For this review, take the finished solid that the model builds, in its own axes (mm). Face numbers are marked on the shaded views. A direction names the side the tool comes from. Round coordinates to 2 decimals unless told otherwise and drop trailing zeros. Write each loop counter-clockwise with the first axis right and the second up, starting at its lowest first coordinate (ties: lowest second). Pieces come first, ordered by that corner, then holes. Notation, with made-up numbers: M 29.5,0.25 L 55.5,0.25 A16 cw 55.5,10.25 Z; hole C -18,27 d5. An arc over 180 degrees is marked long. One line per question, with ' | ' between items.
```python
from build123d import *

# Parameters (mm, degrees)
SKETCH1_W                                       = 140
SKETCH1_H                                       = 30
BOSS_EXTRUDE1_DEPTH                             = 30
SHELL1_T                                        = -5
SKETCH3_W                                       = 5
SKETCH3_H                                       = 20
BOSS_EXTRUDE2_DEPTH                             = 25
SKETCH4_R                                       = 2.5
BOSS_EXTRUDE3_DEPTH                             = 5
SKETCH5_R                                       = 1.5
CUT_EXTRUDE1_DEPTH                              = 20
CUT_EXTRUDE2_DEPTH                              = 152.079449297
CUT_EXTRUDE2_DEPTH_BACK                         = 152.079449297
SKETCH9_R                                       = 5
SKETCH10_W                                      = 140
SKETCH10_H                                      = 5
BOSS_EXTRUDE5_DEPTH                             = 15
SKETCH11_W                                      = 135
SKETCH11_H                                      = 5
CUT_EXTRUDE3_DEPTH                              = 2
FILLET1_R                                       = 2
CSK_FOR_M5_FLAT_HEAD_MACHINE_SCREW1_D           = 5.5
CSK_FOR_M5_FLAT_HEAD_MACHINE_SCREW1_DEPTH       = 20
CSK_FOR_M5_FLAT_HEAD_MACHINE_SCREW1_CSINK_D     = 10.4
CSK_FOR_M5_FLAT_HEAD_MACHINE_SCREW1_CSINK_ANGLE = 90
CSK_FOR_M5_FLAT_HEAD_MACHINE_SCREW1_TIP         = 1.652366702
FILLET2_R                                       = 5


with BuildPart() as part:
    # Sketch1 → Boss-Extrude1 (new body)
    with BuildSketch(Plane(origin=(0, 0, 0), x_dir=(1, 0, 0), z_dir=(0, 1, 0))):
        with Locations((70, 15)):
            Rectangle(SKETCH1_W, SKETCH1_H)
    extrude(amount=BOSS_EXTRUDE1_DEPTH)

    # Shell1
    shell1_openings = [part.faces().sort_by_distance(p)[0] for p in [
        (70, 0, -15),
    ]]
    offset(amount=SHELL1_T, openings=shell1_openings, kind=Kind.INTERSECTION)

    # Sketch3 → Boss-Extrude2 (add)
    with BuildSketch(Plane.XZ.offset(-25)):
        with Locations((52.5, -15)):
            Rectangle(SKETCH3_W, SKETCH3_H)
    extrude(amount=BOSS_EXTRUDE2_DEPTH)

    # Sketch4 → Boss-Extrude3 (add)
    with BuildSketch(Plane(origin=(140, 0, 0), x_dir=(0, 0, -1), z_dir=(1, 0, 0))):
        with Locations(Location((8, 22, 0), (0, 0, 180))):
            Circle(SKETCH4_R)
        with Locations(Location((22, 22, 0), (0, 0, 180))):
            Circle(SKETCH4_R)
        with Locations(Location((8, 8, 0), (0, 0, 180))):
            Circle(SKETCH4_R)
        with Locations(Location((22, 8, 0), (0, 0, 180))):
            Circle(SKETCH4_R)
    extrude(amount=BOSS_EXTRUDE3_DEPTH)

    # Sketch5 → Cut-Extrude1 (cut)
    with BuildSketch(Plane.ZY):
        with Locations((-15, 15)):
            Circle(SKETCH5_R)
    extrude(amount=-CUT_EXTRUDE1_DEPTH, mode=Mode.SUBTRACT)

    # Sketch9 → Cut-Extrude2 (cut, two sides: drawn at the far end of the back side and taken through both)
    with BuildSketch(Plane.XY.offset(-CUT_EXTRUDE2_DEPTH_BACK)):
        with Locations((125, 15)):
            Circle(SKETCH9_R)
    extrude(amount=CUT_EXTRUDE2_DEPTH + CUT_EXTRUDE2_DEPTH_BACK, mode=Mode.SUBTRACT)

    # Sketch10 → Boss-Extrude5 (add)
    with BuildSketch(Plane(origin=(0, 30, 0), x_dir=(1, 0, 0), z_dir=(0, 1, 0))):
        with Locations((70, 17.5)):
            Rectangle(SKETCH10_W, SKETCH10_H)
    extrude(amount=BOSS_EXTRUDE5_DEPTH)

    # Sketch11 → Cut-Extrude3 (cut)
    with BuildSketch(Plane.XY.offset(-15)):
        with Locations((72.5, 37.5)):
            Rectangle(SKETCH11_W, SKETCH11_H)
    extrude(amount=-CUT_EXTRUDE3_DEPTH, mode=Mode.SUBTRACT)

    # Fillet1
    fillet1_edges = [part.edges().sort_by_distance(p)[0] for p in [
        (70, 45, -15),
    ]]
    fillet(fillet1_edges, radius=FILLET1_R)

    # CSK for M5 Flat Head Machine Screw1
    with Locations(Plane.ZY):
        with Locations((-15, 15)):
            CounterSinkHole(CSK_FOR_M5_FLAT_HEAD_MACHINE_SCREW1_D / 2, CSK_FOR_M5_FLAT_HEAD_MACHINE_SCREW1_CSINK_D / 2, depth=CSK_FOR_M5_FLAT_HEAD_MACHINE_SCREW1_DEPTH, counter_sink_angle=CSK_FOR_M5_FLAT_HEAD_MACHINE_SCREW1_CSINK_ANGLE)
            with Locations((0, 0, -(CSK_FOR_M5_FLAT_HEAD_MACHINE_SCREW1_DEPTH + CSK_FOR_M5_FLAT_HEAD_MACHINE_SCREW1_TIP / 2))):  # 118° drill point
                Cone(0, CSK_FOR_M5_FLAT_HEAD_MACHINE_SCREW1_D / 2, CSK_FOR_M5_FLAT_HEAD_MACHINE_SCREW1_TIP, mode=Mode.SUBTRACT)

    # Fillet2
    fillet2_edges = [part.edges().sort_by_distance(p)[0] for p in [
        (70, 30, 0),
    ]]
    fillet(fillet2_edges, radius=FILLET2_R)


solid = part.part
```
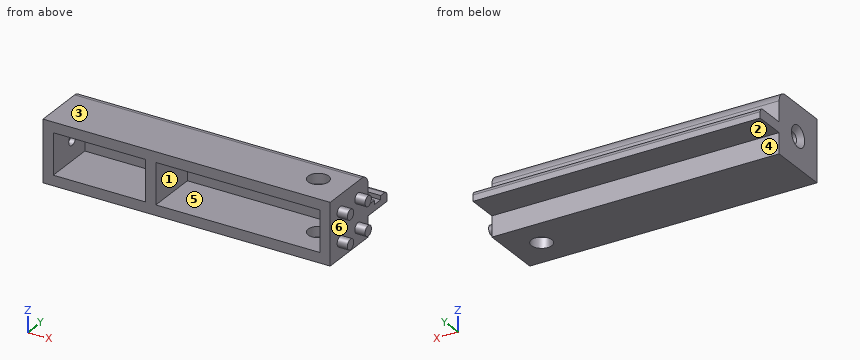
Item 1: Take a section at B-B (x = 125). Write out the cut boundary in (y, z).
Results:
outline: M 0,-30 L 10,-30 L 10,-25 L 0,-25 Z; M 0,-5 L 10,-5 L 10,0 L 0,0 Z; M 20,-30 L 30,-30 L 30,-20 L 45,-20 L 45,-17 A2 ccw 43,-15 L 40,-15 L 40,-17 L 35,-17 L 35,-15 L 30,-15 L 30,-5 A5 ccw 25,0 L 20,0 L 20,-5 L 25,-5 L 25,-25 L 20,-25 Z
Item 2: Mouldability with a two-part tool opening along X and no side actions: class the marked faces 4, 5 and 6 as +X half, -X half, draft (parallel to the pull), parting line (faces both ways), or undercut.
Results:
face 4: draft | face 5: undercut | face 6: +X half
Item 3: Take a section at A-A (y = 15). Write out the cut boundary in (x, z).
Results:
outline: M 0,-30 L 120,-30 L 120,-25 L 55,-25 L 55,-5 L 120,-5 L 120,0 L 0,0 L 0,-9.8 L 2.45,-12.25 L 5,-12.25 L 5,-5 L 50,-5 L 50,-25 L 5,-25 L 5,-17.75 L 2.45,-17.75 L 0,-20.2 Z; M 130,-30 L 140,-30 L 140,0 L 130,0 L 130,-5 L 135,-5 L 135,-25 L 130,-25 Z
Item 4: Take a section at D-D (z = -22). Write out the cut boundary in (x, y).
Results:
outline: M 0,0 L 5,0 L 5,25 L 50,25 L 50,0 L 55,0 L 55,25 L 135,25 L 135,0 L 140,0 L 140,5.5 L 145,5.5 L 145,10.5 L 140,10.5 L 140,19.5 L 145,19.5 L 145,24.5 L 140,24.5 L 140,30 L 0,30 Z
Item 5: Machinability: for the marked faces 1, 2 and 3, which of the approach directions +Z, -Z, +X, -X, +Y, -Y give a long, thin tool a straight path to every point of the face, cutting with its end or side? Answer none if there is none.
Results:
face 1: -Y | face 2: -Z, +X, -X, +Y | face 3: +Z, +X, -X, +Y, -Y
Item 6: Take a section at C-C (y = 4). Write out the cut boundary in (x, z), then the cut area to 3 significant figures.
Results:
outline: M 0,-30 L 140,-30 L 140,0 L 0,0 Z; hole M 5,-25 L 50,-25 L 50,-5 L 5,-5 Z; hole M 55,-25 L 135,-25 L 135,-5 L 55,-5 Z | area: 1,700 mm2
Item 7: Insertion check: pin 1 Ø2.5 at (x, y) = (56, 38.5) entering from +Z; pin 2 Ø3 at (x, z) = (45.5, -10) entering from -Y; pin 3 Ø12 at (y, z) = (35.5, -17.5) entering from +X. Each pin has a flat end and moves straight along its axis. Give the tip position at first contact, or say it passes through.
Results:
pin 1: z = -17 | pin 2: y = 25 | pin 3: x = 140
Item 8: To check wall thickness, follow line 1 along X through (y, z) = (6, -23.75); line 2 along Z through (x, y) = (115.5, 11); line 3 along Y through (x, z) = (125, -26.35). State the ranges of each line that lie inside material, in increasing order. Write a range as from..to.
Results:
line 1: 0..5, 50..55, 135..140 | line 2: -30..-25, -5..0 | line 3: 0..10, 20..30
